The listing builds one solid part. Answer for the finished solid, in the listing's coordinates (mm). Round coordinates to 2 decimals unless told otherwise and drop trailing zeros. Loops run counter-clockwise (first coordinate to the right, second up) from the corner with the lowest first, then second, coordinate; pieces in that order, holes last. Notation, with made-up numbers: M 0,82.25 L 20,82.25 A11 cw 20,91.25 Z; hole C 82,-36 d5. An arc over 180 degrees is marked long. Put each result on its own line as item: value. Start each with the question number.
(1) Section B-B, the plane x = 0 is taken. Determine the outline of the cut face in (y, z), then the cut area to 3 significant figures.
(2) Straight lines are drawn through the part: line 1 (X direction, y = -2.15, z = -4); line 2 (Z direction, x = -10, y = -0.3); line 3 (Y direction, x = 15.5, z = 21). For each, find the intervals that lie inside material, in ascending order.
(3) Section A-A, the plane z = 51 is taken. Determine the outline of the cut face in (x, y).
(4) Flat-ended cylindrical pins translate along their axes: P1, Ø1.5, axis at y = -1.5, z = -32.5, coming from the +X side; P2, Ø2.5, axis at x = 1, y = -1.5, coming from the +Z side. Find the tip coordinate at first contact, or state that the pin passes through.
Autodesk Inventor part; units mm, degrees
ref_plane "YZ Plane" through (0, 0, 0) normal (1, 0, 0) x (0, 1, 0)
ref_plane "XZ Plane" through (0, 0, 0) normal (0, 1, 0) x (-1, 0, 0)
ref_plane "XY Plane" through (0, 0, 0) normal (0, 0, 1) x (1, 0, 0)
sketch "Sketch1" plane through (0, 0, 0) normal (0, 1, 0) x (-1, 0, 0)
  line L0 (-18, -58) -> (18, -58)
  line L1 (18, -58) -> (18, 58)
  line L2 (18, 58) -> (-18, 58)
  line L3 (-18, 58) -> (-18, -58)
  line L4 (-18, -58) -> (18, 58) construction
  line L5 (18, -58) -> (-18, 58) construction
  point P0 (0, 0)
  dimension "d0" = 36
  dimension "d1" = 116
extrude "Extrusion1" add sketch "Sketch1" along normal blind 3
sketch "Sketch2" plane through (0, 0, 0) normal (0, -1, 0) x (1, 0, 0)
  line L0 (15, 55) -> (-15, 55)
  line L1 (-15, 55) -> (-15, -55)
  line L2 (-15, -55) -> (15, -55)
  line L3 (15, -55) -> (15, 55)
  line L4 (15, 55) -> (-15, -55) construction
  line L5 (-15, 55) -> (15, -55) construction
  line L6 (-18, -58) -> (-18, 58)
  line L7 (18, -58) -> (-18, -58)
  point P0 (0, 0)
  dimension "d4" = 3
  dimension "d5" = 3
extrude "Extrusion2" add sketch "Sketch2" along normal blind 3
fillet "Fillet1" radius 2 8 edges at (18, 1.5, 58) (15, -1.5, 55) (-15, -1.5, 55) (-18, 1.5, 58) (15, -1.5, -55) (18, 1.5, -58) (-18, 1.5, -58) (-15, -1.5, -55)
properties part number "module-lid_switch"
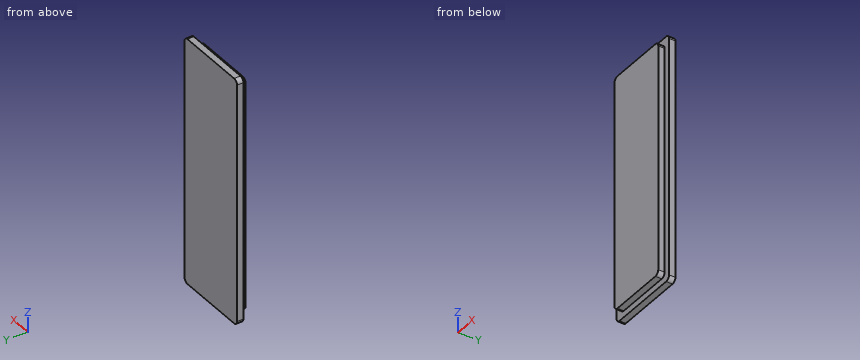
Recorded:
1. outline: M -3,-55 L 0,-55 L 0,-58 L 3,-58 L 3,58 L 0,58 L 0,55 L -3,55 Z
1. area: 678 mm²
2. line 1: x = -15 to 15
2. line 2: z = -55 to 55
2. line 3: y = 0 to 3
3. outline: M -18,0 L -15,0 L -15,-3 L 15,-3 L 15,0 L 18,0 L 18,3 L -18,3 Z
4. P1: stops at x = 15
4. P2: stops at z = 55
